Part model, mm, in its own coordinate system. A direction names the side the tool comes from. Coordinates: 2 decimals unless noted, no trailing zeros. Loops run counter-clockwise (first coordinate to the right, second up) from the corner with the lowest first, then second, coordinate; pieces in that order, holes last. Notation, with made-up numbers: (60.5, 69.5) -> (71.5, 69.5) arc R25 cw to (71.5, 107.5) -> close; hole circle Ø3 at (40, -28.75). An arc over 180 degrees is marked (long way). One line per item, written item: value. Start each with the question number.
Autodesk Inventor part; units mm, degrees
ref_plane "YZ Plane" through (0, 0, 0) normal (1, 0, 0) x (0, 1, 0)
ref_plane "XZ Plane" through (0, 0, 0) normal (0, 1, 0) x (-1, 0, 0)
ref_plane "XY Plane" through (0, 0, 0) normal (0, 0, 1) x (1, 0, 0)
sketch "Sketch1" plane through (0, 0, 0) normal (0, 1, 0) x (-1, 0, 0)
  line L0 (0, 0) -> (-155, 0)
  line L1 (-155, 0) -> (-155, -65)
  line L2 (-155, -65) -> (0, -65)
  line L3 (0, -65) -> (0, 0)
  dimension "d0" = 155
  dimension "d1" = 65
extrude "Extrusion1" add sketch "Sketch1" along normal blind 80
sketch "Sketch2" plane through (0, 80, 0) normal (0, 1, 0) x (1, 0, 0)
  line L0 (155, 0) -> (155, 65)
  line L1 (155, 65) -> (0, 65)
  line L2 (0, 65) -> (0, 0)
  line L3 (0, 0) -> (155, 0)
  line L4 (3, 62) -> (152, 62)
  line L5 (152, 62) -> (152, 3)
  line L6 (152, 3) -> (3, 3)
  line L7 (3, 3) -> (3, 62)
  dimension "d4" = 3
extrude "Extrusion2" cut sketch "Sketch2" against normal blind 77 contours L4 L5 L6 L7
sketch "Sketch3" plane through (0, 0, 0) normal (0, 0, 1) x (1, 0, 0)
  circle A0 centre (28.75, 56.25) radius 12
  circle A1 centre (61.25, 23.75) radius 12
  circle A2 centre (93.75, 56.25) radius 12
  circle A3 centre (126.25, 23.75) radius 12
  point P0 (0, 0)
  dimension "d7" = 24
  dimension "d8" = 24
  dimension "d9" = 24
  dimension "d10" = 24
extrude "Extrusion3" cut sketch "Sketch3" against normal blind 3
sketch "Sketch4" plane through (155, 0, -65) normal (0, 0, -1) x (-1, 0, 0)
  circle A0 centre (28.75, 56.25) radius 12
  circle A1 centre (61.25, 23.75) radius 12
  circle A2 centre (93.75, 56.25) radius 12
  circle A3 centre (126.25, 23.75) radius 12
  point P0 (155, 0)
  dimension "d13" = 24
  dimension "d14" = 24
  dimension "d15" = 24
  dimension "d16" = 24
extrude "Extrusion4" cut sketch "Sketch4" against normal blind 3
sketch "Sketch5" plane through (0, 3, 0) normal (0, 1, 0) x (1, 0, 0)
  line L0 (152, 3) -> (3, 3)
  line L1 (152, 62) -> (152, 3)
  line L2 (3, 62) -> (152, 62)
  line L3 (3, 3) -> (3, 62)
  line L4 (3, 62) -> (12, 62)
  line L5 (12, 62) -> (12, 53)
  line L6 (12, 53) -> (3, 53)
  line L7 (3, 53) -> (3, 62)
  point P0 (0, 0)
  point P1 (3, 57.5)
  point P2 (3, 53)
  dimension "d19" = 9
  dimension "d20" = 9
  dimension "d21" = 0
  dimension "d22" = 0
extrude "Extrusion5" add sketch "Sketch5" along normal blind 77 contours L3 L2 L5 L6
fillet "Fillet1" radius 3 4 edges at (0, 40, 0) (0, 40, -65) (155, 40, -65) (155, 40, 0)
sketch "Sketch8" plane through (0, 80, 0) normal (0, 1, 0) x (1, 0, 0)
  circle A0 centre (7.5, 57.5) radius 2.25
  arc A1 (152, 0) -> (155, 3) centre (152, 3) ccw
  line L0 (155, 3) -> (155, 62)
  arc A2 (155, 62) -> (152, 65) centre (152, 62) ccw
  line L1 (152, 65) -> (3, 65)
  arc A3 (3, 65) -> (0, 62) centre (3, 62) ccw
  line L2 (0, 62) -> (0, 3)
  arc A4 (0, 3) -> (3, 0) centre (3, 3) ccw
  line L3 (3, 0) -> (152, 0)
  line L4 (3, 3) -> (3, 53)
  line L5 (3, 53) -> (12, 53)
  line L6 (12, 53) -> (12, 62)
  line L7 (12, 62) -> (152, 62)
  line L8 (152, 62) -> (152, 3)
  line L9 (152, 3) -> (3, 3)
  point P0 (0, 0)
  dimension "d45" = 4.5
  dimension "d46" = 4.5
  dimension "d47" = 4.5
extrude "Extrusion8" cut sketch "Sketch8" against normal blind 4.5 contours A0
sketch "Sketch9" plane through (7.5, 75.5, -57.5) normal (0, 1, 0) x (1, 0, 0)
  circle A0 centre (0, 0) radius 2.25
  circle A1 centre (0, 0) radius 1.6
  point P0 (-7.5, -57.5)
  dimension "d50" = 3.2
extrude "Extrusion9" cut sketch "Sketch9" against normal blind 2.5 contours A1
pattern_linear "Rectangular Pattern2" count 2 spacing 140 along (1, 0, 0) count 2 spacing -50 along (0, 0, -1) of "Extrusion5", "Extrusion8", "Extrusion9"
fillet "Fillet4" radius 3 4 edges at (12, 41.5, -53) (12, 41.5, -12) (143, 41.5, -53) (143, 41.5, -12)
fillet "Fillet5" radius 2 8 edges at (3, 41.5, -53) (12, 41.5, -62) (3, 41.5, -12) (12, 41.5, -3) (152, 41.5, -53) (143, 41.5, -62) (152, 41.5, -12) (143, 41.5, -3)
properties part number "arcade_box_iteration3"
1) Probe line 1 (X direction, y = 77.8, z = -57.5); line 2 (Z direction, x = 148, y = 22.5); line 3 (Z direction, x = 48, y = 40). List the from-to ranges inside material, lowest first. Write a range as from..to.
2) Pin check, flat tips, straight feed: pin 1 Ø21.5 at (x, y) = (28.75, 23.75) entering from -Z; pin 2 Ø2 at (x, z) = (7.5, -7.5) entering from +Y; pin 3 Ø3 at (x, z) = (57.5, -57) entering from +Y. Stop position of each tip, or through.
3) Slice it at C-C (z = -57.5). Give the cut face in (x, y), then the cut area to 3 significant figures.
4) Tool access for faces 4 (the cylindrical face through (7.292, 74.268, -59.086)), 5 (the cylindrical face through (84.227, 48.948, -1.479)), 6 (the cylindrical face through (138.24, 56.78, -63.52)): list every direction of +Z, -Z, +X, -X, +Y, -Y with a clear straight run to the whole face (end or side of a thin tool).
5) Slice it at A-A (x = 93.75). Give the cut face in (y, z).
6) Pull direction X, two halves, no side cores. Call faces 1 (the cylindrical face through (0.9, 40.56, -64.14)), 2 (the flat face through (79, 39, -65)), 3 (the cylindrical face through (7.21, 77.78, -59.73)): +X half, -X half, draft (parallel to the pull), parting line (faces both ways), or undercut.
7) Slice it at D-D (x = 147.5). Give the cut face in (y, z), then the cut area to 3 significant figures.
Check sheet entries:
1. line 1: x = 0..5.25, 9.75..12, 143..145.25, 149.75..155
1. line 2: z = -65..-53, -12..0
1. line 3: z = -65..-62, -3..0
2. pin 1: stops at z = -3
2. pin 2: stops at y = 73
2. pin 3: stops at y = 3
3. outline: (0, 0) -> (155, 0) -> (155, 80) -> (149.75, 80) -> (149.75, 75.5) -> (149.1, 75.5) -> (149.1, 73) -> (145.9, 73) -> (145.9, 75.5) -> (145.25, 75.5) -> (145.25, 80) -> (143, 80) -> (143, 3) -> (12, 3) -> (12, 80) -> (9.75, 80) -> (9.75, 75.5) -> (9.1, 75.5) -> (9.1, 73) -> (5.9, 73) -> (5.9, 75.5) -> (5.25, 75.5) -> (5.25, 80) -> (0, 80) -> close
3. area: 2,260 mm^2
4. face 4: +Y
4. face 5: +Z
4. face 6: -Z
5. outline: (0, -65) -> (11.75, -65) -> (11.75, -62) -> (3, -62) -> (3, -3) -> (44.25, -3) -> (44.25, 0) -> (0, 0) -> close; (35.75, -65) -> (80, -65) -> (80, -62) -> (35.75, -62) -> close; (68.25, -3) -> (80, -3) -> (80, 0) -> (68.25, 0) -> close
6. face 1: -X half
6. face 2: draft
6. face 3: undercut
7. outline: (0, -65) -> (80, -65) -> (80, -59.75) -> (75.5, -59.75) -> (75.5, -59.1) -> (73, -59.1) -> (73, -55.9) -> (75.5, -55.9) -> (75.5, -55.25) -> (80, -55.25) -> (80, -53) -> (3, -53) -> (3, -12) -> (80, -12) -> (80, -9.75) -> (75.5, -9.75) -> (75.5, -9.1) -> (73, -9.1) -> (73, -5.9) -> (75.5, -5.9) -> (75.5, -5.25) -> (80, -5.25) -> (80, 0) -> (0, 0) -> close
7. area: 1,990 mm^2
